Model file for the job. Use its own axes, mm. Face numbers are marked on the shaded views. A direction names the side the tool comes from. Coordinates: 2 decimals unless noted, no trailing zeros. Order: outer loops, then holes, each group sorted by start corner. A loop starts at its lowest first (then second) coordinate and runs counter-clockwise, first axis right, second up. Notation, with made-up numbers: (30, 44.5) -> (75, 44.5) arc R16 ccw to (75, 69.5) -> close; hole circle Ø1 at (81, 57.25). An arc over 180 degrees is marked (long way). Write item = value, one per line. Start each with the question number.
Q1. Mould opens along Z. For the marked faces 1, 2, 3 and 4 say: +Z half, -Z half, draft (parallel to the pull), parting line (faces both ways), or undercut.
Q2. Cut at A-A, the plane x = -1. List the corners of the cut face in (y, z).
Q3. Cut at B-B, the plane z = 7.35. List the corners of the cut face in (x, y).
Q4. Wall check: line 1 (X direction, y = 5, z = -17.5); line 2 (Z direction, x = -5.5, y = 6); line 3 (X direction, y = 2.5, z = -7.35). Give the ranges that are in metal, low to high. Write a range as from..to.
Q5. 3-axis set-ups, long thin cutter, end or side, ignore diameter. For the marked faces 5, 6, 7, 8 and 9: which of +Z, -Z, +X, -X, +Y, -Y reach the whole face in a straight line?
Q6. Cut at D-D, the plane z = -32. List the corners of the cut face in (x, y), plus the area to 3 significant figures.
Q7. Cut at C-C, the plane y = 5.25. Give the number of separate pieces and of enclosed holes in the cut face, plus the area to 3 significant figures.
Q8. Flat gauge pins, fed straight in: pin 1 (1 mm diameter, centred on y = 6, z = -23, fed in from -X); pin 2 (1.5 mm diameter, centred on x = 2, y = 6.5, fed in from +Z) (3 decimals); pin 3 (3 mm diameter, centred on x = 3, z = -30, fed in from +Y). Where does each tip first touch, or does it go through?
from build123d import *

# Parameters (mm, degrees)
SKETCH1_W           = 19
SKETCH1_H           = 54
BOSS_EXTRUDE4_DEPTH = 2
SKETCH1_8_R         = 1.96
SKETCH1_8_W         = 19
SKETCH1_8_H         = 54
SKETCH1_8_W_2       = 15
SKETCH1_8_H_2       = 50
BOSS_EXTRUDE7_DEPTH = 10


with BuildPart() as part:
    # Sketch1 → Boss-Extrude4 (new body)
    with BuildSketch(Plane(origin=(0, 0, 0), x_dir=(1, 0, 0), z_dir=(0, 1, 0))):
        with BuildLine():
            ThreePointArc((-12.939793146, 39.228116436), (-20.958488329, 28.375411428), (-17.576524537, 15.31237199))
            ThreePointArc((-17.576524537, 15.31237199), (-19.723741965, 7.787946982), (-20.482290695, 0))
            ThreePointArc((-20.482290695, 0), (-19.723741965, -7.787946982), (-17.576524537, -15.31237199))
            ThreePointArc((-17.576524537, -15.31237199), (-20.958488329, -28.375411428), (-12.939793146, -39.228116436))
            ThreePointArc((-12.939793146, -39.228116436), (-6.193274653, -38.828364827), (0, -36.123062219))
            ThreePointArc((0, -36.123062219), (6.193274653, -38.828364827), (12.939793146, -39.228116436))
            ThreePointArc((12.939793146, -39.228116436), (20.958488329, -28.375411428), (17.576524537, -15.31237199))
            ThreePointArc((17.576524537, -15.31237199), (19.723741965, -7.787946982), (20.482290695, 0))
            ThreePointArc((20.482290695, 0), (19.723741965, 7.787946982), (17.576524537, 15.31237199))
            ThreePointArc((17.576524537, 15.31237199), (20.958488329, 28.375411428), (12.939793146, 39.228116436))
            ThreePointArc((12.939793146, 39.228116436), (6.193274653, 38.828364827), (0, 36.123062219))
            ThreePointArc((0, 36.123062219), (-6.193274653, 38.828364827), (-12.939793146, 39.228116436))
        make_face()
        Rectangle(SKETCH1_W, SKETCH1_H, mode=Mode.SUBTRACT)
    extrude(amount=BOSS_EXTRUDE4_DEPTH)

    # Sketch1_8 → Boss-Extrude7 (add)
    with BuildSketch(Plane(origin=(0, 0, 0), x_dir=(1, 0, 0), z_dir=(0, 1, 0))):
        with BuildLine():
            ThreePointArc((0, 47.123463385), (11.906709568, 49.134588213), (23.603104913, 46.133139939))
            ThreePointArc((23.603104913, 46.133139939), (28.130450168, 42.466846104), (28.423306673, 36.648530145))
            ThreePointArc((28.423306673, 36.648530145), (31.044925166, 25.293928807), (28.336730948, 13.959664864))
            ThreePointArc((28.336730948, 13.959664864), (29.774673681, 7.044655791), (30.282467524, 0))
            ThreePointArc((30.282467524, 0), (29.774673681, -7.044655791), (28.336730948, -13.959664864))
            ThreePointArc((28.336730948, -13.959664864), (31.044925166, -25.293928807), (28.423306673, -36.648530145))
            ThreePointArc((28.423306673, -36.648530145), (28.130450168, -42.466846104), (23.603104913, -46.133139939))
            ThreePointArc((23.603104913, -46.133139939), (11.906709568, -49.134588213), (0, -47.123463385))
            ThreePointArc((0, -47.123463385), (-11.906709568, -49.134588213), (-23.603104913, -46.133139939))
            ThreePointArc((-23.603104913, -46.133139939), (-28.130450168, -42.466846104), (-28.423306673, -36.648530145))
            ThreePointArc((-28.423306673, -36.648530145), (-31.044925166, -25.293928807), (-28.336730948, -13.959664864))
            ThreePointArc((-28.336730948, -13.959664864), (-29.774673681, -7.044655791), (-30.282467524, 0))
            ThreePointArc((-30.282467524, 0), (-29.774673681, 7.044655791), (-28.336730948, 13.959664864))
            ThreePointArc((-28.336730948, 13.959664864), (-31.044925166, 25.293928807), (-28.423306673, 36.648530145))
            ThreePointArc((-28.423306673, 36.648530145), (-28.130450168, 42.466846104), (-23.603104913, 46.133139939))
            ThreePointArc((-23.603104913, 46.133139939), (-11.906709568, 49.134588213), (0, 47.123463385))
        make_face()
        with Locations((24.5, 7.35)):
            Circle(SKETCH1_8_R, mode=Mode.SUBTRACT)
        with Locations((24.5, -7.35)):
            Circle(SKETCH1_8_R, mode=Mode.SUBTRACT)
        with Locations((21.760807675, -39.229711143)):
            Circle(SKETCH1_8_R, mode=Mode.SUBTRACT)
        with Locations((-24.5, -7.35)):
            Circle(SKETCH1_8_R, mode=Mode.SUBTRACT)
        with Locations((-24.5, 7.35)):
            Circle(SKETCH1_8_R, mode=Mode.SUBTRACT)
        with Locations((-21.760807675, 39.229711143)):
            Circle(SKETCH1_8_R, mode=Mode.SUBTRACT)
        with Locations((-21.760807675, -39.229711143)):
            Circle(SKETCH1_8_R, mode=Mode.SUBTRACT)
        with Locations((21.760807675, 39.229711143)):
            Circle(SKETCH1_8_R, mode=Mode.SUBTRACT)
        with BuildLine():
            ThreePointArc((0, 36.123062219), (-6.193274653, 38.828364827), (-12.939793146, 39.228116436))
            ThreePointArc((-12.939793146, 39.228116436), (-20.958488329, 28.375411428), (-17.576524537, 15.31237199))
            ThreePointArc((-17.576524537, 15.31237199), (-19.723741965, 7.787946982), (-20.482290695, 0))
            ThreePointArc((-20.482290695, 0), (-19.723741965, -7.787946982), (-17.576524537, -15.31237199))
            ThreePointArc((-17.576524537, -15.31237199), (-20.958488329, -28.375411428), (-12.939793146, -39.228116436))
            ThreePointArc((-12.939793146, -39.228116436), (-6.193274653, -38.828364827), (0, -36.123062219))
            ThreePointArc((0, -36.123062219), (6.193274653, -38.828364827), (12.939793146, -39.228116436))
            ThreePointArc((12.939793146, -39.228116436), (20.958488329, -28.375411428), (17.576524537, -15.31237199))
            ThreePointArc((17.576524537, -15.31237199), (19.723741965, -7.787946982), (20.482290695, 0))
            ThreePointArc((20.482290695, 0), (19.723741965, 7.787946982), (17.576524537, 15.31237199))
            ThreePointArc((17.576524537, 15.31237199), (20.958488329, 28.375411428), (12.939793146, 39.228116436))
            ThreePointArc((12.939793146, 39.228116436), (6.193274653, 38.828364827), (0, 36.123062219))
        make_face(mode=Mode.SUBTRACT)
        Rectangle(SKETCH1_8_W, SKETCH1_8_H)
        Rectangle(SKETCH1_8_W_2, SKETCH1_8_H_2, mode=Mode.SUBTRACT)
    extrude(amount=BOSS_EXTRUDE7_DEPTH)


solid = part.part
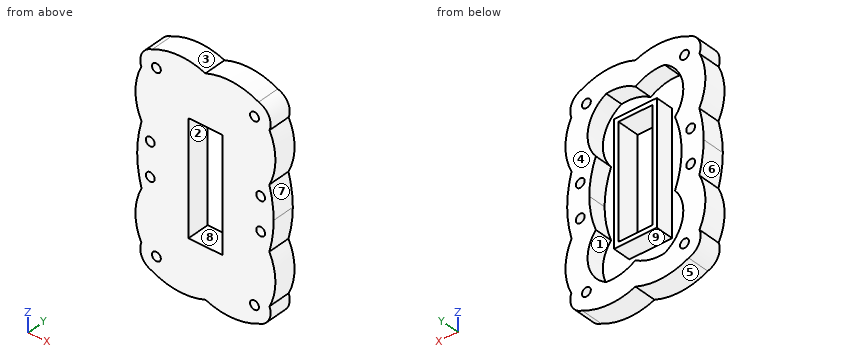
Here are the results:
q1.face_1 = undercut
q1.face_2 = undercut
q1.face_3 = +Z half
q1.face_4 = draft
q2.outline = (0, -47.5) -> (10, -47.5) -> (10, -36.75) -> (2, -36.75) -> (2, -27) -> (10, -27) -> (10, -25) -> (0, -25) -> close; (0, 25) -> (10, 25) -> (10, 27) -> (2, 27) -> (2, 36.75) -> (10, 36.75) -> (10, 47.5) -> (0, 47.5) -> close
q3.outline = (-29.73, 0) -> (-26.46, 0) -> (-26.46, 10) -> (-29.73, 10) -> close; (-22.54, 0) -> (-7.5, 0) -> (-7.5, 10) -> (-9.5, 10) -> (-9.5, 2) -> (-19.8, 2) -> (-19.8, 10) -> (-22.54, 10) -> close; (7.5, 0) -> (22.54, 0) -> (22.54, 10) -> (19.8, 10) -> (19.8, 2) -> (9.5, 2) -> (9.5, 10) -> (7.5, 10) -> close; (26.46, 0) -> (29.73, 0) -> (29.73, 10) -> (26.46, 10) -> close
q4.line_1 = -29.79..-19.11, -9.5..-7.5, 7.5..9.5, 19.11..29.79
q4.line_2 = -48.69..-38.65, -27..-25, 25..27, 38.65..48.69
q4.line_3 = -29.73..-26.46, -22.54..-19.8, -9.5..-7.5, 7.5..9.5, 19.8..22.54, 26.46..29.73
q5.face_5 = -Z, +Y, -Y
q5.face_6 = -X, +Y, -Y
q5.face_7 = +X, +Y, -Y
q5.face_8 = +Y, -Y
q5.face_9 = +Y
q6.outline = (-30.17, 0) -> (30.17, 0) -> (30.17, 10) -> (19.78, 10) -> (19.78, 2) -> (-19.78, 2) -> (-19.78, 10) -> (-30.17, 10) -> close
q6.area = 287 mm²
q7.separate_pieces = 2
q7.enclosed_holes = 10
q7.area = 2,830 mm²
q8.pin_1 = -30.97
q8.pin_2 = 48.055
q8.pin_3 = 2
